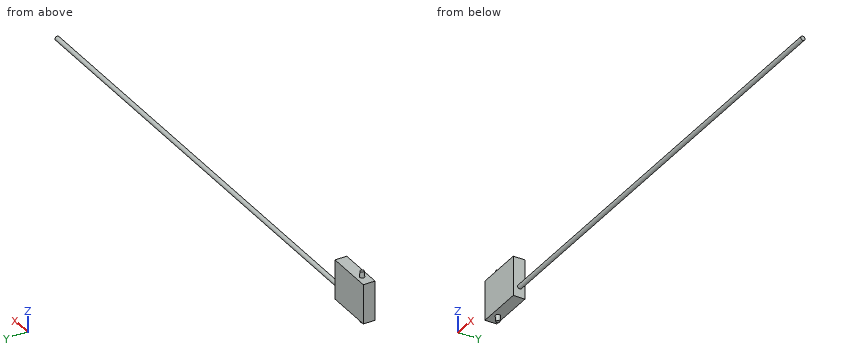
```python
from build123d import *

# Parameters (mm, degrees)
SKETCH1_W           = 25.4
SKETCH1_H           = 21.59
BOSS_EXTRUDE1_DEPTH = 6.35
SKETCH2_R           = 1.27
BOSS_EXTRUDE2_DEPTH = 3.175
BOSS_EXTRUDE2_TAPER = 5
SKETCH3_R           = 1.169045739
BOSS_EXTRUDE3_DEPTH = 254


with BuildPart() as part:
    # Sketch1 → Boss-Extrude1 (new body)
    with BuildSketch(Plane(origin=(0, 0, 0), x_dir=(1, 0, 0), z_dir=(0, 1, 0))):
        Rectangle(SKETCH1_W, SKETCH1_H)
    extrude(amount=BOSS_EXTRUDE1_DEPTH)

    # Sketch2 → Boss-Extrude2 (add)
    with BuildSketch(Plane.XY.offset(10.795)):
        with Locations((-6.35, 3.175)):
            Circle(SKETCH2_R)
    boss_extrude2 = extrude(amount=BOSS_EXTRUDE2_DEPTH, taper=BOSS_EXTRUDE2_TAPER)

    # Mirror1: Boss-Extrude2 across plane
    add(boss_extrude2.mirror(Plane.XY))

    # Sketch3 → Boss-Extrude3 (add)
    with BuildSketch(Plane(origin=(12.7, 0, 0), x_dir=(0, 0, -1), z_dir=(1, 0, 0))):
        with Locations((4.956387533, 3.55)):
            Circle(SKETCH3_R)
    extrude(amount=BOSS_EXTRUDE3_DEPTH)


solid = part.part
```
Here's how the part is built. I have some questions about the finished solid (model axes, mm). Give positions to 0.01 mm unless a question says otherwise; leave off trailing zeros. Order: outer loops, then holes, each group sorted by start corner. A loop starts at its lowest first (then second) coordinate and runs counter-clockwise, first axis right, second up. Notation, with made-up numbers: (62.25, 41.25) -> (121.25, 41.25) arc R29 ccw to (121.25, 80.25) -> close; hole circle Ø8 at (69, -29). An arc over 180 degrees is marked (long way). Use CSV: the item, a comma, the result in double quotes. Start each with the question number.
Item 1: Suppose I cut it at B-B (x = 87). List the corners of the cut face in (y, z) for me.
Item 2: If I drill on probe 1 along X at (y, z) = (4.75, 8.5); probe 2 along Y at (x, z) = (240, -4.75); probe 3 along Z at (x, y) = (186, 3.25), over which ranges is the centre line in solid material (lowest first)? Write a range as [from, to].
Item 3: Suppose I cut it at A-A (z = 4.5). List the corners of the cut face in (x, y) for me.
Item 4: I'm going to push flat-ended pins straight in: P1, Ø2, axis at x = 52.5, z = -4.5, coming from the +Y side; P2, Ø3, axis at x = -1.5, y = 5, coming from the +Z side (3 decimals); P3, Ø1.5, axis at y = 2.5, z = -9.5, coming from the +X side. Where does each tip first touch, or does it pass through?
Answer block:
1,outline,"circle Ø2.34 at (3.55, -4.96)"
2,probe 1,"x = [-12.7, 12.7]"
2,probe 2,"y = [2.4, 4.7]"
2,probe 3,"z = [-6.09, -3.83]"
3,outline,"(-12.7, 0) -> (12.7, 0) -> (12.7, 6.35) -> (-12.7, 6.35) -> close"
4,P1,"stops at y = 4.72"
4,P2,"stops at z = 10.795"
4,P3,"stops at x = 12.7"
